The listing builds one solid part. Answer for the finished solid, in the listing's coordinates (mm). A direction names the side the tool comes from. Coordinates: 2 decimals unless noted, no trailing zeros. Order: outer loops, then holes, each group sorted by start corner. A loop starts at its lowest first (then second) coordinate and runs counter-clockwise, first axis right, second up.
```python
from build123d import *

# Parameters (mm, degrees)
BOSS_EXTRUDE1_DEPTH = 170
SKETCH3_R           = 75
SKETCH3_R_2         = 62.5
BOSS_EXTRUDE2_DEPTH = 75
SKETCH4_W           = 150
SKETCH4_H           = 150
BOSS_EXTRUDE3_DEPTH = 225
CUT_EXTRUDE6_DEPTH  = 225
SKETCH6_R           = 62.5
BOSS_EXTRUDE4_DEPTH = 75
BOSS_EXTRUDE5_START = -10
SKETCH7_R           = 67.5
SKETCH7_R_2         = 62.5
BOSS_EXTRUDE5_DEPTH = 10
SKETCH8_W           = 10
SKETCH8_H           = 12.412745851


with BuildPart() as part:
    # Sketch2 → Boss-Extrude1 (new body)
    with BuildSketch(Plane.XY):
        Polygon((-40.398264296, 30.238450413), (-20.398264296, 30.238450413), (-20.398264296, -139.761549587), (149.601735704, -139.761549587), (149.601735704, -159.761549587), (-40.398264296, -159.761549587), align=None)
    extrude(amount=-BOSS_EXTRUDE1_DEPTH)

    # Sketch3 → Boss-Extrude2 (add)
    with BuildSketch(Plane.ZY.offset(40.398264296)):
        with Locations((-85.93846623, -54.761549587)):
            Circle(SKETCH3_R)
        with Locations((-85.93846623, -54.761549587)):
            Circle(SKETCH3_R_2, mode=Mode.SUBTRACT)
    extrude(amount=BOSS_EXTRUDE2_DEPTH)

    # Sketch4 → Boss-Extrude3 (add)
    with BuildSketch(Plane(origin=(-20.398264296, 0, 0), x_dir=(0, 0, -1), z_dir=(1, 0, 0))):
        with Locations((85, -54.761549587)):
            Rectangle(SKETCH4_W, SKETCH4_H)
    extrude(amount=BOSS_EXTRUDE3_DEPTH)

    # Sketch5 → Cut-Extrude6 (cut)
    with BuildSketch(Plane(origin=(204.601735704, 0, 0), x_dir=(0, 0, -1), z_dir=(1, 0, 0))):
        with BuildLine():
            Line((35, 20.238450413), (10, 20.238450413))
            Line((10, 20.238450413), (10, -4.761549587))
            ThreePointArc((10, -4.761549587), (27.67766953, 2.560780883), (35, 20.238450413))
        make_face()
        with BuildLine():
            ThreePointArc((35, -129.761549587), (27.67766953, -112.083880057), (10, -104.761549587))
            Line((10, -104.761549587), (10, -129.761549587))
            Line((10, -129.761549587), (35, -129.761549587))
        make_face()
        with BuildLine():
            ThreePointArc((160, -104.761549587), (142.32233047, -112.083880057), (135, -129.761549587))
            Line((135, -129.761549587), (160, -129.761549587))
            Line((160, -129.761549587), (160, -104.761549587))
        make_face()
        with BuildLine():
            Line((160, 20.238450413), (135, 20.238450413))
            ThreePointArc((135, 20.238450413), (142.32233047, 2.560780883), (160, -4.761549587))
            Line((160, -4.761549587), (160, 20.238450413))
        make_face()
    extrude(amount=-CUT_EXTRUDE6_DEPTH, mode=Mode.SUBTRACT)

    # Sketch6 → Boss-Extrude4 (add)
    with BuildSketch(Plane.XZ.offset(159.761549587)):
        with Locations((64.601735704, -85)):
            Circle(SKETCH6_R)
    extrude(amount=BOSS_EXTRUDE4_DEPTH)

    # Sketch7 → Boss-Extrude5 (add)
    with BuildSketch(Plane.XZ.offset(234.761549587).offset(BOSS_EXTRUDE5_START)):
        with Locations((64.601735704, -85)):
            Circle(SKETCH7_R)
        with Locations((64.601735704, -85)):
            Circle(SKETCH7_R_2, mode=Mode.SUBTRACT)
    extrude(amount=BOSS_EXTRUDE5_DEPTH)

    # Sketch8 → Cut-Revolve1 (revolve, cut)
    with BuildSketch(Plane.XZ.offset(54.761549587), mode=Mode.PRIVATE) as cut_revolve1_sk:
        with Locations((-45.398264296, -24.644839156)):
            Rectangle(SKETCH8_W, SKETCH8_H)
    revolve(cut_revolve1_sk.sketch.rotate(Axis((-115.398264296, -54.761549587, -85.93846623), (1, 0, 0)), 180), axis=Axis((-115.398264296, -54.761549587, -85.93846623), (1, 0, 0)), mode=Mode.SUBTRACT)


solid = part.part
```
(1) For faces 1 (the face through (93.68, -112.28, -27.87)), 2 (the face through (-77.37, -83.49, -16.66)), 3 (the face through (93.68, -111.89, -142.52)), 4 (the face through (91, -55, -160)), 5 (the face through (84, -224.762, -145)), determine the directions among +Z, -Z, +X, -X, +Y, -Y from which every point of the face is accessible in a straight line to the end or side of a thin tool.
(2) Each of these flat-tipped pins is pushed along its axis until it touches: pin 1 Ø12 at (y, z) = (-52.5, -32) entering from -X; pin 2 Ø1 at (x, z) = (134, -118.5) entering from -Y; pin 3 Ø10 at (y, z) = (-148.5, -100.5) entering from +X; pin 4 Ø3 at (x, y) = (-64.5, -132.5) entering from +Z. Where does it stop, or does it pass through?
(3) Consider line 1 (Y direction, x = 82, z = -49); line 2 (Y direction, x = 121.5, z = -131); line 3 (Z direction, x = 100, y = -75.5). Determine where each line is inside the solid, lowest interval first.
(4) Find section B-B (x = 106.5). Write down the section's boundary in (y, z), and give its area (3 significant figures).
(5) The mould has two halves that part along Y. Classify faces 6 (the face through (100.889, -229.692, -28.084)), 7 (the face through (91, -129.762, -84)), 8 (the face through (91, 20.238, -84)): released by +Y, released by -Y, zero draft, split by the parting line, or undercut.
(6) Find section C-C (y = -47.5). Write down the section's boundary in (x, z), and give its area (3 significant figures).
Findings below:
1. face 1: +Z, +X
1. face 2: -X
1. face 3: -Z, +X
1. face 4: -Z, +X, +Y
1. face 5: none
2. pin 1: stops at x = -40.4
2. pin 2: stops at y = -159.76
2. pin 3: stops at x = 149.6
2. pin 4: passes through
3. line 1: y = -234.76 to -139.76, -129.76 to 20.24
3. line 2: y = -159.76 to -139.76, -129.76 to 20.24
3. line 3: z = -160 to -10
4. outline: (-234.76, -137.92) - (-224.76, -137.92) - (-224.76, -131.38) - (-159.76, -131.38) - (-159.76, -170) - (-139.76, -170) - (-139.76, 0) - (-159.76, 0) - (-159.76, -38.62) - (-224.76, -38.62) - (-224.76, -32.08) - (-234.76, -32.08) - close; (-129.76, -135) arc R25 cw to (-104.76, -160) - (-4.76, -160) arc R25 cw to (20.24, -135) - (20.24, -35) arc R25 cw to (-4.76, -10) - (-104.76, -10) arc R25 cw to (-129.76, -35) - close
4. area: 31,000 mm2
5. face 6: zero draft
5. face 7: undercut
5. face 8: released by +Y
6. outline: (-115.4, -160.59) - (-40.4, -160.59) - (-40.4, -170) - (-20.4, -170) - (-20.4, -160) - (204.6, -160) - (204.6, -10) - (-20.4, -10) - (-20.4, 0) - (-40.4, 0) - (-40.4, -11.29) - (-115.4, -11.29) - (-115.4, -23.86) - (-50.4, -23.86) - (-50.4, -18.83) - (-40.4, -18.83) - (-40.4, -153.05) - (-50.4, -153.05) - (-50.4, -148.02) - (-115.4, -148.02) - close
6. area: 38,900 mm2
